Geometry check sheet. Reference: the model listing, model coordinates, mm. A direction names the side the tool comes from. Give positions to 0.01 mm unless a question says otherwise; leave off trailing zeros. Order: outer loops, then holes, each group sorted by start corner. A loop starts at its lowest first (then second) coordinate and runs counter-clockwise, first axis right, second up. Notation, with made-up numbers: M 10,53 L 52,53 A16 ccw 52,80 Z; hole C -4.75,-11.5 d3. An arc over 180 degrees is marked long. Answer as CSV lines item,"result".
from build123d import *

# Parameters (mm, degrees)
SKETCH1_R           = 1.7859375
SKETCH1_R_2         = 1.5875
BOSS_EXTRUDE1_DEPTH = 0.8128


with BuildPart() as part:
    # Sketch1 → Boss-Extrude1 (new body)
    with BuildSketch(Plane.XY):
        with BuildLine():
            Line((17.374031657, -2.38125), (17.374031657, 10.31875))
            ThreePointArc((17.374031657, 10.31875), (14.199031657, 13.49375), (11.024031657, 10.31875))
            Line((11.024031657, 10.31875), (11.024031657, 9.128125))
            ThreePointArc((11.024031657, 9.128125), (9.977853691, 6.602427966), (7.452156657, 5.55625))
            Line((7.452156657, 5.55625), (7.14374999, 5.55625))
            ThreePointArc((7.14374999, 5.55625), (4.618052962, 6.602427969), (3.571875, 9.128125))
            ThreePointArc((3.571875, 9.128125), (-0.713207259, 12.628071631), (-3.287058429, 7.730434799))
            ThreePointArc((-3.287058429, 7.730434799), (-3.061446655, 5.68510334), (-4.001636336, 3.854714088))
            ThreePointArc((-4.001636336, 3.854714088), (-5.113201992, -2.17418478), (0, -5.55625))
            Line((0, -5.55625), (12.611531657, -5.55625))
            Line((12.611531657, -5.55625), (12.611531657, -6.36905))
            Line((12.611531657, -6.36905), (15.786531657, -6.36905))
            Line((15.786531657, -6.36905), (15.786531657, -5.130880657))
            ThreePointArc((15.786531657, -5.130880657), (16.948662314, -3.96875), (17.374031657, -2.38125))
        make_face()
        Circle(SKETCH1_R, mode=Mode.SUBTRACT)
        with Locations((14.199031657, -1.5875)):
            Circle(SKETCH1_R_2, mode=Mode.SUBTRACT)
        with Locations((0, 9.128125)):
            Circle(SKETCH1_R, mode=Mode.SUBTRACT)
        with Locations((14.199031657, 9.525)):
            Circle(SKETCH1_R_2, mode=Mode.SUBTRACT)
    extrude(amount=BOSS_EXTRUDE1_DEPTH)


solid = part.part
(1) Section check D-D on x = 14.5. Enter the section's corners in (y, z).
The answers:
outline,"M -6.37,0 L -3.15,0 L -3.15,0.81 L -6.37,0.81 Z; M -0.03,0 L 7.97,0 L 7.97,0.81 L -0.03,0.81 Z; M 11.08,0 L 13.48,0 L 13.48,0.81 L 11.08,0.81 Z"
(2) Draft check along Y on faces 1 (the face through (14.2, -6.369, 0.4)), 2 (the face through (15.787, -5.8, 0.4)), 3 (the face through (-0.387, 7.385, 0.401)). Enter one of: +Y half, -Y half, draft (parallel to the pull), parting line (faces both ways), or undercut.
The answers:
face 1,"-Y half"
face 2,"draft"
face 3,"undercut"
(3) Material ranges on line 1 (Y direction, x = 14.25, z = 0.65); line 2 (X direction, y = 9.5, z = 0.6); line 3 (X direction, y = -1.5, z = 0.25), recorded low to high.
The answers:
line 1,"y = -6.37 to -3.17, 0 to 7.94, 11.11 to 13.49"
line 2,"x = -3.55 to -1.75, 1.75 to 3.55, 11.02 to 12.61, 15.79 to 17.37"
line 3,"x = -5.35 to -0.97, 0.97 to 12.61, 15.78 to 17.37"
(4) Tool access check on faces 4 (the face through (-1.784, 0.079, 0.401)), 5 (the face through (10.005, 6.63, 0.401)), 6 (the face through (6.2, -5.556, 0.4)). Record the directions out of +Z, -Z, +X, -X, +Y, -Y that give a thin tool (end or side, any length) a straight path to the whole face; none if there is none.
The answers:
face 4,"+Z, -Z"
face 5,"+Z, -Z, +Y"
face 6,"+Z, -Z, -X, -Y"
(5) Section check A-A on x = -1.5. Enter the section's corners in (y, z).
The answers:
outline,"M -5.35,0 L -0.97,0 L -0.97,0.81 L -5.35,0.81 Z; M 0.97,0 L 8.16,0 L 8.16,0.81 L 0.97,0.81 Z; M 10.1,0 L 12.37,0 L 12.37,0.81 L 10.1,0.81 Z"
(6) Section check B-B on y = 8.5. Enter the section's corners in (x, z), then the cut area to 3 significant figures.
The answers:
outline,"M -3.52,0 L -1.67,0 L -1.67,0.81 L -3.52,0.81 Z; M 1.67,0 L 3.63,0 L 3.63,0.81 L 1.67,0.81 Z; M 10.97,0 L 12.99,0 L 12.99,0.81 L 10.97,0.81 Z; M 15.41,0 L 17.37,0 L 17.37,0.81 L 15.41,0.81 Z"
area,"6.32 mm2"
(7) Section check C-C on z = 0.5. State how many separate pieces and enclosed holes the cut face has, then the cut area to 3 significant figures.
The answers:
separate pieces,"1"
enclosed holes,"4"
area,"303 mm2"
